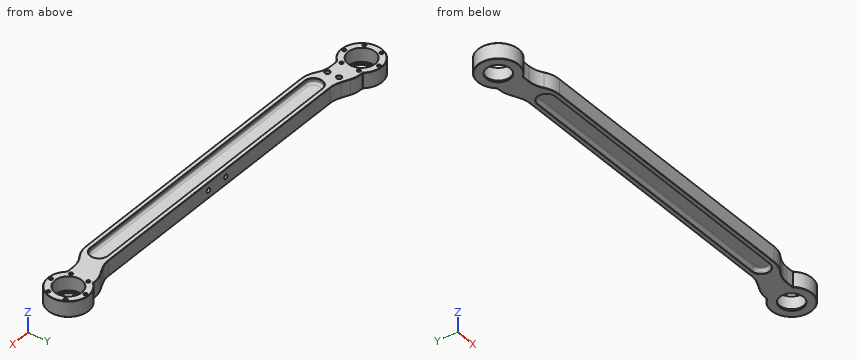
from build123d import *

# Parameters (mm, degrees)
EXTRUDE_1_DEPTH     = 13.5
CUT_EXTRUDE_1_DEPTH = 8.5
SKETCH_3_R          = 4
CUT_EXTRUDE_2_DEPTH = 15
SKETCH_6_R          = 23.5
CUT_EXTRUDE_3_DEPTH = 24
SKETCH_6_3_R        = 2.5
CUT_EXTRUDE_4_DEPTH = 15
SKETCH_6_4_R        = 20.5
CUT_EXTRUDE_5_DEPTH = 379.001653436
FILLET_1_R          = 4
SKETCH_7_R          = 4
CUT_EXTRUDE_6_DEPTH = 15
CHAMFER_1_SIZE      = 0.5


with BuildPart() as part:
    # Sketch 1 → Extrude 1 (new, symmetric)
    with BuildSketch(Plane.XY):
        with BuildLine():
            Line((-252.817923204, 45), (252.817923204, 45))
            ThreePointArc((252.817923204, 45), (262.557705831, 46.06667968), (271.835744982, 49.216149583))
            Line((271.835744982, 49.216149583), (285.944523165, 55.795180897))
            ThreePointArc((285.944523165, 55.795180897), (295.222562316, 58.944650801), (304.962344943, 60.01133048))
            Line((304.962344943, 60.01133048), (308.2, 60.01133048))
            ThreePointArc((308.2, 60.01133048), (369.999999218, 37.492602678), (308.190486763, 15))
            Line((308.190486763, 15), (295, 15))
            ThreePointArc((295, 15), (282.009618943, 13.084219849), (270.125314072, 7.5))
            ThreePointArc((270.125314072, 7.5), (258.241009201, 1.915780151), (245.250628145, 0))
            Line((245.250628145, 0), (-245.250628145, 0))
            ThreePointArc((-245.250628145, 0), (-258.241009201, 1.915780151), (-270.125314072, 7.5))
            ThreePointArc((-270.125314072, 7.5), (-282.009618943, 13.084219849), (-295, 15))
            Line((-295, 15), (-308.190486763, 15))
            ThreePointArc((-308.190486763, 15), (-369.999999218, 37.492602678), (-308.2, 60.01133048))
            Line((-308.2, 60.01133048), (-304.962344943, 60.01133048))
            ThreePointArc((-304.962344943, 60.01133048), (-295.222562316, 58.944650801), (-285.944523165, 55.795180897))
            Line((-285.944523165, 55.795180897), (-271.835744982, 49.216149583))
            ThreePointArc((-271.835744982, 49.216149583), (-262.557705831, 46.06667968), (-252.817923204, 45))
        make_face()
    extrude(amount=EXTRUDE_1_DEPTH, both=True)

    # Sketch 2 → Cut-Extrude 1 (cut)
    with BuildSketch(Plane.XY.offset(13.5)):
        with BuildLine():
            Line((-245, 37.5), (245, 37.5))
            ThreePointArc((245, 37.5), (260, 22.5), (245, 7.5))
            Line((245, 7.5), (-245, 7.5))
            ThreePointArc((-245, 7.5), (-260, 22.5), (-245, 37.5))
        make_face()
    cut_extrude_1 = extrude(amount=-CUT_EXTRUDE_1_DEPTH, mode=Mode.SUBTRACT)

    # Mirror 1: Cut-Extrude 1 across plane
    add(cut_extrude_1.mirror(Plane.XY), mode=Mode.SUBTRACT)

    # Sketch 3 → Cut-Extrude 2 (cut)
    with BuildSketch(Plane(origin=(0, 45, 0), x_dir=(1, 0, 0), z_dir=(0, 1, 0))):
        with Locations(Location((-15, 0, 0), (0, 0, 180))):
            Circle(SKETCH_3_R)
        with Locations(Location((25, 0, 0), (0, 0, 180))):
            Circle(SKETCH_3_R)
    extrude(amount=-CUT_EXTRUDE_2_DEPTH, mode=Mode.SUBTRACT)

    # Sketch 6 → Cut-Extrude 3 (cut)
    with BuildSketch(Plane.XY.offset(13.5)):
        with Locations((335, 37.5)):
            Circle(SKETCH_6_R)
        with Locations(Location((-335, 37.5, 0), (0, 0, 180))):
            Circle(SKETCH_6_R)
    extrude(amount=-CUT_EXTRUDE_3_DEPTH, mode=Mode.SUBTRACT)

    # Sketch 6_3 → Cut-Extrude 4 (cut)
    with BuildSketch(Plane.XY.offset(13.5)):
        with Locations((335, 67.5)):
            Circle(SKETCH_6_3_R)
        with Locations((360.980762114, 52.5)):
            Circle(SKETCH_6_3_R)
        with Locations((360.980762114, 22.5)):
            Circle(SKETCH_6_3_R)
        with Locations((335, 7.5)):
            Circle(SKETCH_6_3_R)
        with Locations((309.019237886, 22.5)):
            Circle(SKETCH_6_3_R)
        with Locations((309.019237886, 52.5)):
            Circle(SKETCH_6_3_R)
        with Locations(Location((-309.019237886, 52.5, 0), (0, 0, 180))):
            Circle(SKETCH_6_3_R)
        with Locations(Location((-309.019237886, 22.5, 0), (0, 0, 180))):
            Circle(SKETCH_6_3_R)
        with Locations(Location((-335, 7.5, 0), (0, 0, 180))):
            Circle(SKETCH_6_3_R)
        with Locations(Location((-360.980762114, 22.5, 0), (0, 0, 180))):
            Circle(SKETCH_6_3_R)
        with Locations(Location((-360.980762114, 52.5, 0), (0, 0, 180))):
            Circle(SKETCH_6_3_R)
        with Locations(Location((-335, 67.5, 0), (0, 0, 180))):
            Circle(SKETCH_6_3_R)
    extrude(amount=-CUT_EXTRUDE_4_DEPTH, mode=Mode.SUBTRACT)

    # Sketch 6_4 → Cut-Extrude 5 (cut, through all)
    with BuildSketch(Plane.XY.offset(13.5)):
        with Locations((-335, 37.5)):
            Circle(SKETCH_6_4_R)
        with Locations((335, 37.5)):
            Circle(SKETCH_6_4_R)
    extrude(amount=-CUT_EXTRUDE_5_DEPTH, mode=Mode.SUBTRACT)

    # Fillet 1
    fillet_1_edges = [part.edges().sort_by_distance(p)[0] for p in [
        (-260, 22.5, 5),
        (0, 37.5, 5),
        (260, 22.5, 5),
        (0, 7.5, 5),
        (-260, 22.5, -5),
        (0, 7.5, -5),
        (260, 22.5, -5),
        (0, 37.5, -5),
    ]]
    fillet(fillet_1_edges, radius=FILLET_1_R)

    # Sketch 7 → Cut-Extrude 6 (cut)
    with BuildSketch(Plane.XY.offset(13.5)):
        with Locations((-280, 40)):
            Circle(SKETCH_7_R)
        with Locations((-280, 20)):
            Circle(SKETCH_7_R)
    extrude(amount=-CUT_EXTRUDE_6_DEPTH, mode=Mode.SUBTRACT)

    # Chamfer 1
    chamfer_1_edges = [part.edges().sort_by_distance(p)[0] for p in [
        (306.519237886, 22.5, 13.5),
        (306.519237886, 52.5, 13.5),
        (332.5, 67.5, 13.5),
        (-332.5, 67.5, 13.5),
        (-358.480762114, 52.5, 13.5),
        (-358.480762114, 22.5, 13.5),
        (-306.519237886, 52.5, 13.5),
        (-306.519237886, 22.5, 13.5),
        (332.5, 7.5, -1.5),
        (332.5, 7.5, 13.5),
        (358.480762114, 22.5, -1.5),
        (358.480762114, 22.5, 13.5),
        (358.480762114, 52.5, -1.5),
        (358.480762114, 52.5, 13.5),
        (-332.5, 7.5, 13.5),
        (-262.557705831, 46.06667968, 13.5),
        (-278.890134073, 52.50566524, 13.5),
        (278.890134073, 52.50566524, -13.5),
        (295.222562316, 58.944650801, -13.5),
        (-284, 40, 13.5),
        (-284, 20, 13.5),
        (306.581172471, 60.01133048, -13.5),
        (369.999999218, 37.492602678, -13.5),
        (301.595243382, 15, -13.5),
        (282.009618943, 13.084219849, -13.5),
        (258.241009201, 1.915780151, -13.5),
        (0, 0, -13.5),
        (-258.241009201, 1.915780151, -13.5),
        (-295.222562316, 58.944650801, 13.5),
        (-282.009618943, 13.084219849, -13.5),
        (-301.595243382, 15, -13.5),
        (-369.999999218, 37.492602678, -13.5),
        (-306.581172471, 60.01133048, -13.5),
        (-295.222562316, 58.944650801, -13.5),
        (-278.890134073, 52.50566524, -13.5),
        (-262.557705831, 46.06667968, -13.5),
        (0, 45, -13.5),
        (262.557705831, 46.06667968, -13.5),
        (-306.581172471, 60.01133048, 13.5),
        (-369.999999218, 37.492602678, 13.5),
        (-301.595243382, 15, 13.5),
        (-282.009618943, 13.084219849, 13.5),
        (-258.241009201, 1.915780151, 13.5),
        (0, 0, 13.5),
        (258.241009201, 1.915780151, 13.5),
        (262.557705831, 46.06667968, 13.5),
        (282.009618943, 13.084219849, 13.5),
        (-260, 22.5, 13.5),
        (0, 7.5, 13.5),
        (260, 22.5, 13.5),
        (0, 37.5, 13.5),
        (301.595243382, 15, 13.5),
        (369.999999218, 37.492602678, 13.5),
        (306.581172471, 60.01133048, 13.5),
        (-260, 22.5, -13.5),
        (0, 7.5, -13.5),
        (260, 22.5, -13.5),
        (0, 37.5, -13.5),
        (295.222562316, 58.944650801, 13.5),
        (278.890134073, 52.50566524, 13.5),
        (0, 45, 13.5),
    ]]
    chamfer(chamfer_1_edges, length=CHAMFER_1_SIZE)


solid = part.part
Here's how the part is built. I have some questions about the finished solid (model axes, mm). Round coordinates to 2 decimals unless told otherwise and drop trailing zeros. Order: outer loops, then holes, each group sorted by start corner. A loop starts at its lowest first (then second) coordinate and runs counter-clockwise, first axis right, second up. Notation, with made-up numbers: M -16,-26.5 L 27,-26.5 A23 ccw 27,-0.5 Z; hole C 52,85 d8. An arc over 180 degrees is marked long. One line per question, with ' | ' between items.
1) I need wall thicknesses on line 1 (Y direction, x = -107.5, z = 10); line 2 (Y direction, x = -225, z = -8); line 3 (X direction, y = 33.5, z = -7). Which ranges of each line are inside material? Lowest first, please.
Checked values:
line 1: y = 0 to 7.5, 37.5 to 45 | line 2: y = 0 to 7.63, 37.37 to 45 | line 3: x = -369.77 to -358.16, -311.84 to -254.39, 254.39 to 311.84, 358.16 to 369.77
2) Imagine slicing it at A-A, the plane x = 37. Write out the boundary of the cut face in (y, z), plus the area to 3 significant figures.
Checked values:
outline: M 0,-13 L 0.5,-13.5 L 7,-13.5 L 7.5,-13 L 7.5,-9 A4 cw 11.5,-5 L 33.5,-5 A4 cw 37.5,-9 L 37.5,-13 L 38,-13.5 L 44.5,-13.5 L 45,-13 L 45,13 L 44.5,13.5 L 38,13.5 L 37.5,13 L 37.5,9 A4 cw 33.5,5 L 11.5,5 A4 cw 7.5,9 L 7.5,13 L 7,13.5 L 0.5,13.5 L 0,13 Z | area: 718 mm²
3) I'm going to push flat-ended pins straight in: pin 1 Ø1.2 at (x, z) = (38, 11.5) entering from +Y; pin 2 Ø14 at (x, y) = (326, 40.5) entering from +Z; pin 3 Ø8 at (x, y) = (-15, 23.5) entering from -Z; pin 4 Ø4 at (y, z) = (37.5, -5.5) entering from +X. Where does each tip first touch, or does it pass through?
Checked values:
pin 1: stops at y = 45 | pin 2: passes through | pin 3: stops at z = -5 | pin 4: stops at x = 370
